```python
from build123d import *

# Parameters (mm, degrees)
F_4_40_TAPPED_HOLE1_D               = 2.2606
F_4_40_TAPPED_HOLE1_DEPTH           = 7.62
F_4_40_TAPPED_HOLE1_TIP             = 0.679152758
F_4_40_TAPPED_HOLE1_ON_FACE_2_D     = 2.2606
F_4_40_TAPPED_HOLE1_ON_FACE_2_DEPTH = 7.62
F_4_40_TAPPED_HOLE1_ON_FACE_2_TIP   = 0.679152758
F_4_40_TAPPED_HOLE1_ON_FACE_3_D     = 2.2606
F_4_40_TAPPED_HOLE1_ON_FACE_3_DEPTH = 7.62
F_4_40_TAPPED_HOLE1_ON_FACE_3_TIP   = 0.679152758
F_4_40_TAPPED_HOLE1_ON_FACE_4_D     = 2.2606
F_4_40_TAPPED_HOLE1_ON_FACE_4_DEPTH = 7.62
F_4_40_TAPPED_HOLE1_ON_FACE_4_TIP   = 0.679152758


with BuildPart() as part:
    # Sketch2 → Revolve1 (revolve)
    with BuildSketch(Plane(origin=(0, 0, 0), x_dir=(0, 0, -1), z_dir=(1, 0, 0))):
        Polygon((-17.399, 30.1371), (-11.049, 30.1371), (-11.049, 28.8925), (-8.636, 28.8925), (-8.636, 30.1371), (-4.826, 30.1371), (-4.826, 28.8925), (-2.413, 28.8925), (-2.413, 30.1371), (0, 30.1371), (0, 21.5011), (-11.049, 21.5011), (-11.049, 21.2471), (-17.399, 21.2471), align=None)
    revolve(axis=Axis((0, 0, 0), (0, 0, 1)))

    # #4-40 Tapped Hole1
    with Locations(Plane(origin=(0, -30.1371, 14.224), x_dir=(-1, 0, 0), z_dir=(0, -1, 0))):
        with Locations((0, 0)):
            Hole(F_4_40_TAPPED_HOLE1_D / 2, depth=F_4_40_TAPPED_HOLE1_DEPTH)
            with Locations((0, 0, -(F_4_40_TAPPED_HOLE1_DEPTH + F_4_40_TAPPED_HOLE1_TIP / 2))):  # 118° drill point
                Cone(0, F_4_40_TAPPED_HOLE1_D / 2, F_4_40_TAPPED_HOLE1_TIP, mode=Mode.SUBTRACT)

    # #4-40 Tapped Hole1 on face 2
    with Locations(Plane(origin=(30.1371, 0, 14.224), x_dir=(0, 0, 1), z_dir=(1, 0, 0))):
        with Locations((0, 0)):
            Hole(F_4_40_TAPPED_HOLE1_ON_FACE_2_D / 2, depth=F_4_40_TAPPED_HOLE1_ON_FACE_2_DEPTH)
            with Locations((0, 0, -(F_4_40_TAPPED_HOLE1_ON_FACE_2_DEPTH + F_4_40_TAPPED_HOLE1_ON_FACE_2_TIP / 2))):  # 118° drill point
                Cone(0, F_4_40_TAPPED_HOLE1_ON_FACE_2_D / 2, F_4_40_TAPPED_HOLE1_ON_FACE_2_TIP, mode=Mode.SUBTRACT)

    # #4-40 Tapped Hole1 on face 3
    with Locations(Plane(origin=(-30.1371, 0, 14.224), x_dir=(0, 0, -1), z_dir=(-1, 0, 0))):
        with Locations((0, 0)):
            Hole(F_4_40_TAPPED_HOLE1_ON_FACE_3_D / 2, depth=F_4_40_TAPPED_HOLE1_ON_FACE_3_DEPTH)
            with Locations((0, 0, -(F_4_40_TAPPED_HOLE1_ON_FACE_3_DEPTH + F_4_40_TAPPED_HOLE1_ON_FACE_3_TIP / 2))):  # 118° drill point
                Cone(0, F_4_40_TAPPED_HOLE1_ON_FACE_3_D / 2, F_4_40_TAPPED_HOLE1_ON_FACE_3_TIP, mode=Mode.SUBTRACT)

    # #4-40 Tapped Hole1 on face 4
    with Locations(Plane(origin=(0, 30.1371, 14.224), x_dir=(0, 0, 1), z_dir=(0, 1, 0))):
        with Locations((0, 0)):
            Hole(F_4_40_TAPPED_HOLE1_ON_FACE_4_D / 2, depth=F_4_40_TAPPED_HOLE1_ON_FACE_4_DEPTH)
            with Locations((0, 0, -(F_4_40_TAPPED_HOLE1_ON_FACE_4_DEPTH + F_4_40_TAPPED_HOLE1_ON_FACE_4_TIP / 2))):  # 118° drill point
                Cone(0, F_4_40_TAPPED_HOLE1_ON_FACE_4_D / 2, F_4_40_TAPPED_HOLE1_ON_FACE_4_TIP, mode=Mode.SUBTRACT)

    # Mirror1: part across plane


with BuildPart() as part_1:
    add(part.part)
    add(part.part.mirror(Plane(origin=(0, 30.1371, 0), x_dir=(1, 0, 0), z_dir=(0, 0, -1))))


solid = part_1.part
```
For this review, take the finished solid that the model builds, in its own axes (mm). A direction names the side the tool comes from. Coordinates: 2 decimals unless noted, no trailing zeros. Answer as a JSON object with one key per item and string values. Group by question number.
1. The part is to be moulded in two halves that separate along Z. For faces 6 (the flat face through (-21, -6, -17.399)), 7 (the conical face through (21.956, -0.059, -14.411)), 8 (the cylindrical face through (29.42, -6.53, 6.7)), say which applies: pulls with the +Z half, pulls with the -Z half, needs draft (parallel to the pull), parting line crosses it, or undercut.
2. Clearance check with flat-ended pins moving along their axes: P1, Ø8, axis at y = 2.5, z = 7.5, coming from the +X side; P2, Ø18, axis at x = 2.5, y = -9.5, coming from the +Z side; P3, Ø1, axis at y = -14.5, z = 6, coming from the +X side; P4, Ø1.4, axis at y = 0, z = 14.224, coming from the -X side. State where each tip first meets the part, or that it passes through.
3. For faces 1 (the flat face through (-21, -6, 17.399)), 2 (the cylindrical face through (-26.274, -0.05, -13.095)), 3 (the cylindrical face through (26.27, 0.43, -13.18)), 4 (the flat face through (29, 2, -11.049)), 5 (the cylindrical face through (29.42, -6.53, -6.7)), list the 3-axis set-ups (+Z, -Z, +X, -X, +Y, -Y) from which the entire face can be reached by the end or side of a thin tool; tool diameter is ignored.
4. We need section A-A on x = 26. Give the number of separate pieces and of enclosed holes in the cut face, then the cut area to 3 significant figures.
5. For probe 1 along Z at (x, y) = (0, 25.75); probe 2 along Z at (x, y) = (25, -16); probe 3 along Y at (x, z) = (0, -8.5), list the stretches that pass through material, from the lowest coordinate up.
Final values:
{
 "1": {"face 6": "pulls with the -Z half", "face 7": "undercut", "face 8": "needs draft"},
 "2": {"P1": "x = 30.14", "P2": "through", "P3": "x = 26.69", "P4": "x = -22.26"},
 "3": {"face 1": "+Z, +X, -X, +Y, -Y", "face 2": "-X", "face 3": "+X", "face 4": "none", "face 5": "+Z, -Z"},
 "4": {"separate pieces": "1", "enclosed holes": "2", "area": "1,000 mm²"},
 "5": {"probe 1": "-17.4 to -15.35, -13.09 to 13.09, 15.35 to 17.4", "probe 2": "-17.4 to -11.05, -8.64 to -4.83, -2.41 to 2.41, 4.83 to 8.64, 11.05 to 17.4", "probe 3": "-30.14 to -21.5, 21.5 to 30.14"}
}
